Source: CAD feature listing. Evaluate the final solid. Frame: model axes, mm. A direction names the side the tool comes from. Give positions to 0.01 mm unless a question says otherwise; leave off trailing zeros. Order: outer loops, then holes, each group sorted by start corner. A loop starts at its lowest first (then second) coordinate and runs counter-clockwise, first axis right, second up. Notation, with made-up numbers: (6.25, 12.25) -> (47.25, 12.25) arc R25 cw to (47.25, 26.25) -> close; hole circle Ø10 at (51, -26). An arc over 180 degrees is marked (long way). Answer in a Markdown table with one row per item.
```python
from build123d import *

# Parameters (mm, degrees)
F1_DEPTH = 30
F3_D     = 6.5
F4_R     = 5
F5_R     = 1


with BuildPart() as f1:
    # F0 (on Front) → F1 (new body)
    with BuildSketch(Plane.XZ):
        Polygon((50.5, 0), (0, 0), (-50.5, 0), (-50.5, 103), (-41.288837, 103), (-39.095837, 103), (-50.997918, 114.902082), (-52.2, 113.7), (-43.2, 104.7), (-52.2, 104.7), (-52.2, -1.7), (0, -1.7), (52.2, -1.7), (52.2, 104.7), (43.2, 104.7), (52.2, 113.7), (50.997918, 114.902082), (39.095837, 103), (41.288837, 103), (50.5, 103), align=None)
    extrude(amount=F1_DEPTH)

    # F3 (through all)
    with Locations(Plane.XY):
        with Locations((32.25, -15), (-32.25, -15)):
            Hole(F3_D / 2)

    # F4
    f4_edges = [f1.edges().sort_by_distance(p)[0] for p in [
        (-51.598959, 0, 114.301041),
        (-51.598959, -30, 114.301041),
        (51.598959, 0, 114.301041),
        (51.598959, -30, 114.301041),
    ]]
    fillet(f4_edges, radius=F4_R)

    # F5
    f5_edges = [f1.edges().sort_by_distance(p)[0] for p in [
        (52.2, -15, 104.7),
        (-39.095837, -15, 103),
        (-52.2, -15, 104.7),
        (-50.5, -15, 0),
        (52.2, -15, -1.7),
        (39.095837, -15, 103),
        (50.5, -15, 0),
        (-52.2, -15, -1.7),
    ]]
    fillet(f5_edges, radius=F5_R)


solid = f1.part
```
(1) Access query for faces 4 (the flat face through (45.972, -14.79, 109.876)), 5 (the flat face through (-47.8, -14.8, 109.3)), 6 (the flat face through (47.6, -14.8, 109.1)), 7 (the flat face through (-46, -15, 103)). Directions: +Z, -Z, +X, -X, +Y, -Y. A direction counts if a zero-diameter tool reaches every point of the face in a straight line with its end or side. Return the directions, or none.
A:
| item | result |
|---|---|
| face 4 | +Z, +Y, -Y |
| face 5 | -X, +Y, -Y |
| face 6 | +X, +Y, -Y |
| face 7 | +Y, -Y |
(2) Section query D-D (y = -22.5). Return the cut outline in (x, z).
A:
| item | result |
|---|---|
| outline | (-52.2, -0.7) arc R1 ccw to (-51.2, -1.7) -> (51.2, -1.7) arc R1 ccw to (52.2, -0.7) -> (52.2, 103.7) arc R1 ccw to (51.2, 104.7) -> (43.2, 104.7) -> (52.2, 113.7) -> (51, 114.9) -> (40.8, 104.71) arc R1 ccw to (41.51, 103) -> (50.5, 103) -> (50.5, 1) arc R1 cw to (49.5, 0) -> (-49.5, 0) arc R1 cw to (-50.5, 1) -> (-50.5, 103) -> (-41.51, 103) arc R1 ccw to (-40.8, 104.71) -> (-51, 114.9) -> (-52.2, 113.7) -> (-43.2, 104.7) -> (-51.2, 104.7) arc R1 ccw to (-52.2, 103.7) -> close |
(3) Section query B-B (y = -15). Give the number of separate pieces and of enclosed holes in the cut face, plus the area to 3 significant figures.
A:
| item | result |
|---|---|
| separate pieces | 3 |
| enclosed holes | 0 |
| area | 591 mm^2 |
(4) Ray query, probe 1 along Y at (x, z) = (32.25, -0.35); probe 2 along X at (y, z) = (-18.75, 19); probe 3 along Z at (x, y) = (-10, -5.5). Return the intervals inside material, ascending.
A:
| item | result |
|---|---|
| probe 1 | y = -30 to -18.25, -11.75 to 0 |
| probe 2 | x = -52.2 to -50.5, 50.5 to 52.2 |
| probe 3 | z = -1.7 to 0 |
(5) First-contact query: pin 1 Ø6.5 at (x, y) = (-46, -11) entering from +Z; pin 2 Ø6.5 at (x, y) = (47.5, -21.5) entering from +Z. Flat tips, straight axial feed; report the tip coordinate or a pass-through.
A:
| item | result |
|---|---|
| pin 1 | stops at z = 113.15 |
| pin 2 | stops at z = 114.65 |
(6) Section query C-C (x = -32.25). Return the cut outline in (y, z).
A:
| item | result |
|---|---|
| outline | (-30, -1.7) -> (-18.25, -1.7) -> (-18.25, 0) -> (-30, 0) -> close; (-11.75, -1.7) -> (0, -1.7) -> (0, 0) -> (-11.75, 0) -> close |
(7) Section query A-A (z = 34.5). Return the cut outline in (x, y).
A:
| item | result |
|---|---|
| outline | (-52.2, -30) -> (-50.5, -30) -> (-50.5, 0) -> (-52.2, 0) -> close; (50.5, -30) -> (52.2, -30) -> (52.2, 0) -> (50.5, 0) -> close |
(8) Pull-direction query (Z, two-part tool) for faces 1 (the cylindrical face through (-50.544, -1.426, 113.229)), 2 (the flat face through (50.5, -15, 53)), 3 (the flat face through (-51, 0, 59)); classes: +Z half, -Z half, draft (parallel to the pull), parting line (faces both ways), or undercut.
A:
| item | result |
|---|---|
| face 1 | +Z half |
| face 2 | undercut |
| face 3 | draft |
